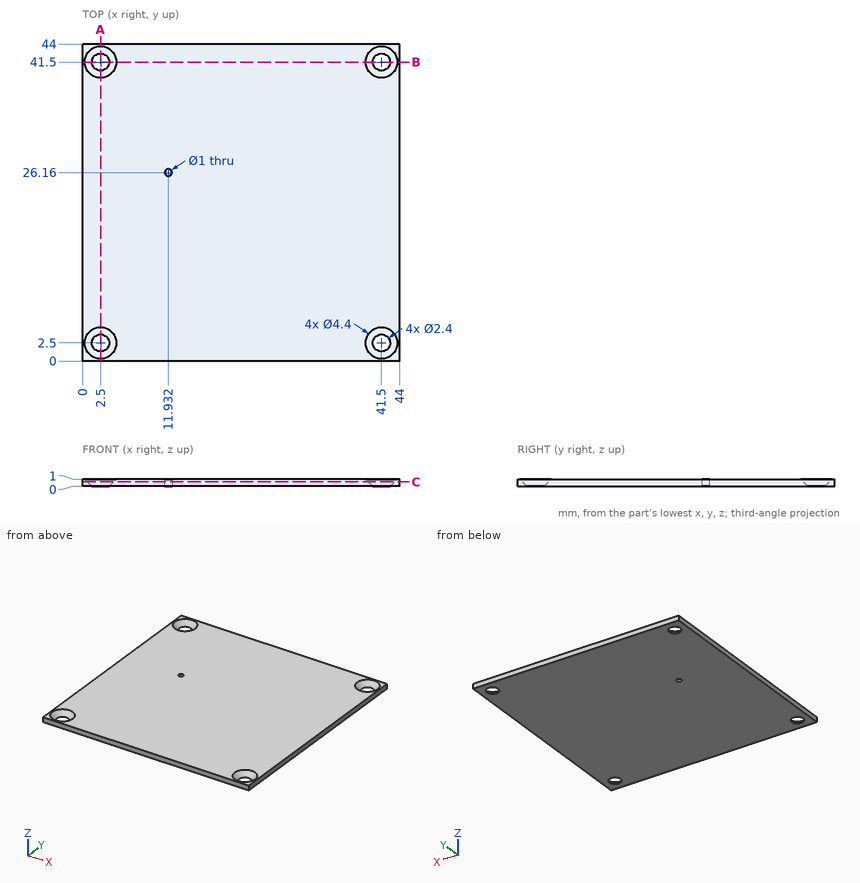
Can you work these out from the drawing? Everything is in mm from the part's minimum corner. Give positions to 0.01 mm unless a question says otherwise; leave off trailing zeros. Loops run counter-clockwise (first coordinate to the right, second up) from the corner with the lowest first, then second, coordinate; pieces in that order, holes last. Notation, with made-up numbers: M 1.5,11 L 17.5,11 A21 ccw 17.5,29 Z; hole C 35.25,1 d6. An arc over 180 degrees is marked long. Put each result on its own line as item: value. Start each with the question number.
(1) Will this pin go through, and if not, where does the flat tip stop? pin 1 Ø6 at (x, y) = (26.5, 35) entering from -Z.
(2) I need wall thicknesses on line 1 along Y through (x, z) = (41, 0.7) (1 decimal); line 2 along Z through (x, y) = (42.5, 40); line 3 along Z through (x, y) = (4, 41). Which ranges of each line are inside material? Lowest first, please. Write a range as [from, to].
(3) I want a section at C-C on z = 0.6. Please give me the cut outline in (x, y).
(4) I want a section at A-A on x = 2.5. Please give me the cut outline in (y, z).
Answer block:
1. pin 1: z = 0
2. line 1: [0, 0.7], [4.3, 39.7], [43.3, 44]
2. line 2: [0, 0.6]
2. line 3: [0, 0.38]
3. outline: M 0,0 L 44,0 L 44,44 L 0,44 Z; hole C 2.5,2.5 d3.6; hole C 2.5,41.5 d3.6; hole C 11.93,26.16 d1; hole C 41.5,2.5 d3.6; hole C 41.5,41.5 d3.6
4. outline: M 0,0 L 1.3,0 L 0.3,1 L 0,1 Z; M 3.7,0 L 40.3,0 L 39.3,1 L 4.7,1 Z; M 42.7,0 L 44,0 L 44,1 L 43.7,1 Z
